Design review of the part shown in the three views and the two pictorial views. Dimensions are in mm from the part's minimum x, y and z. Give positions to 0.01 mm unless a question says otherwise; leave off trailing zeros. Loops run counter-clockwise (first coordinate to the right, second up) from the corner with the lowest first, then second, coordinate; pieces in that order, holes last. Notation, with made-up numbers: (64, 81.5) - (98, 81.5) arc R26 cw to (98, 115.5) - close; hole circle Ø5 at (33.25, 58). An arc over 180 degrees is marked (long way). Return JSON: item names as keys, results as strings. Group by question number.
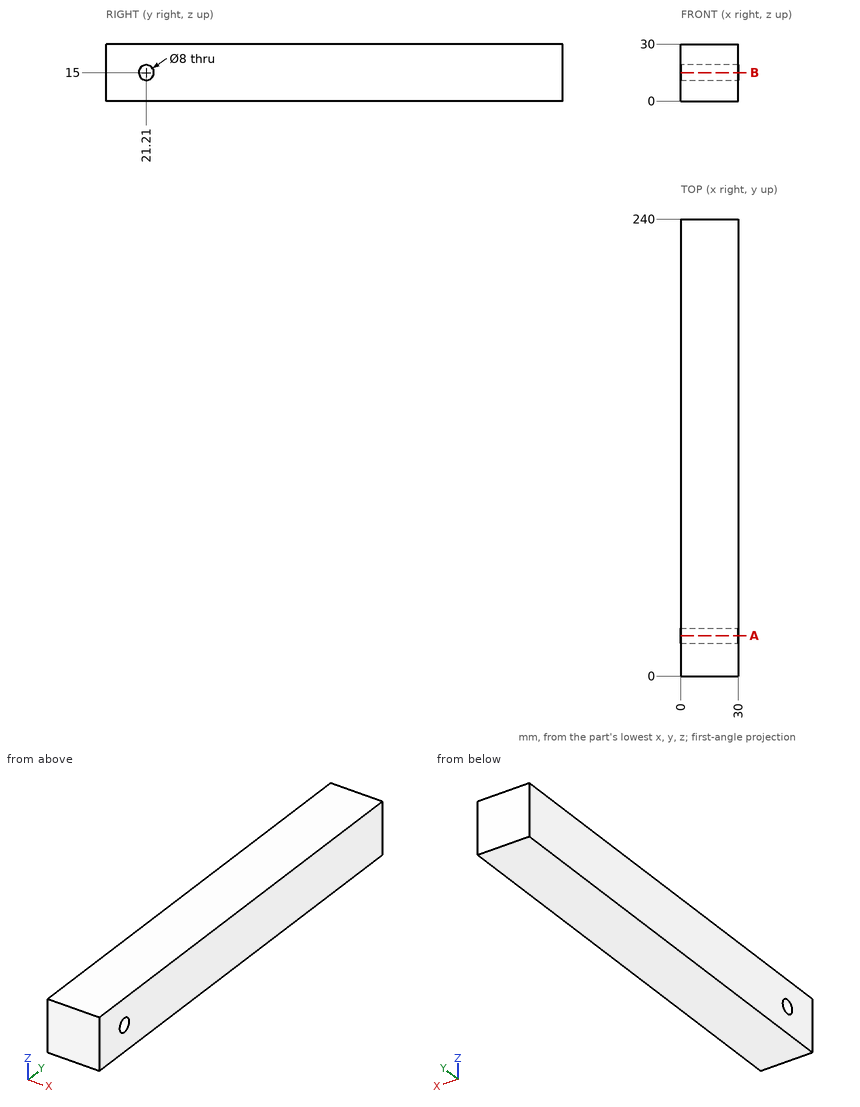
Item 1: Take a section at B-B (z = 15). State the section outline as (x, y) points.
Item 2: For L1, parallel to Y at x = 7, z = 15; L2, parallel to Y at x = 24, z = 13, list the stretches that pass through material, from the lowest coordinate up. Write a range as from..to.
Item 3: Take a section at A-A (y = 21.21). State the section outline as (x, z) points, then the cut area to 3 significant figures.
Item 4: For P1, Ø13, axis at y = 21.21, z = 15, coming from the +X side, flat-tipped, find the tip position at first contact; note if it passes through.
Check sheet entries:
{
 "1": {"outline": "(0, 0) - (30, 0) - (30, 17.21) - (0, 17.21) - close; (0, 25.21) - (30, 25.21) - (30, 240) - (0, 240) - close"},
 "2": {"L1": "y = 0..17.21, 25.21..240", "L2": "y = 0..17.75, 24.67..240"},
 "3": {"outline": "(0, 0) - (30, 0) - (30, 11) - (0, 11) - close; (0, 19) - (30, 19) - (30, 30) - (0, 30) - close", "area": "660 mm^2"},
 "4": {"P1": "stops at x = 30"}
}
